from build123d import *

# Parameters (mm, degrees)
PAD_DEPTH       = 9.5
PAD001_DEPTH    = 9.5
SKETCH002_R     = 2.1
PAD002_DEPTH    = 3
POCKET_DEPTH    = 7
POCKET001_DEPTH = 7.3


with BuildPart() as part:
    # Sketch → Pad (new body, symmetric)
    with BuildSketch(Plane.YZ):
        Polygon((-9.4638496319, 12.9847787924), (0, 13.8127583485), (9.4638496319, 14.6407379046), (11.8731622478, 15.1748696522), (20.8002421453, 18.4240610138), (29.7273220428, 21.6732523754), (31.9162958532, 22.8127600156), (39.698240274, 28.2617361609), (47.4801846947, 33.7107123063), (49.7744904401, 30.4341041291), (34.2106015986, 19.5361518385), (31.0954026161, 17.9144818922), (13.2412428211, 11.416099169), (9.8124726029, 10.6559591122), (-9.1152266609, 9), (-12.6239030908, 9.1531921213), (-31.335250398, 12.452507497), (-34.6847225392, 13.5085920065), (-51.9045704929, 21.5383389795), (-50.2140974459, 25.1635701277), (-41.604173469, 21.1486966411), (-32.9942494922, 17.1338231546), (-30.6406576873, 16.391738509), (-21.2849840337, 14.7420808212), (-11.9293103801, 13.0924231333), align=None)
    extrude(amount=PAD_DEPTH, both=True)

    # Sketch001 → Pad001 (join)
    with BuildSketch(Plane.YZ):
        with BuildLine():
            Line((-32.3771396349, 6.543661009), (-30.6406576873, 16.391738509))
            Line((-30.6406576873, 16.391738509), (-32.9942494922, 17.1338231546))
            Line((-32.9942494922, 17.1338231546), (-37.2204319887, 8.0707452278))
            add(Edge.make_bspline(
                [(-37.2204319887, 8.0707452278), (-39.0096730727, 4.2337052069), (-40, 3), (-45, 3)],
                knots=[0, 0, 0, 0, 1, 1, 1, 1], degree=3))
            Line((-45, 3), (-45, 0))
            Line((-45, 0), (-35, 0))
            Line((-35, 0), (-32.3771396349, 6.543661009))
        make_face()
        Polygon((-13.6657925125, 3.2443456659), (-11.9293103801, 13.0924231333), (-9.4638496319, 12.9847787924), (-8.5922920505, 3.0228318249), (-8.5922920505, 0), (-13.6657925125, 0), align=None)
        Polygon((15.2933760081, 5.777947931), (11.8731622478, 15.1748696522), (9.4638496319, 14.6407379046), (10.3354072218, 4.6787909379), (10.3354072218, 0), (15.2933760081, 0), align=None)
        with BuildLine():
            Line((37.6520787719, 14.6212525652), (31.9162958532, 22.8127600156))
            Line((31.9162958532, 22.8127600156), (29.7273220428, 21.6732523754))
            Line((29.7273220428, 21.6732523754), (33.1475397634, 12.2763320956))
            Line((33.1475397634, 12.2763320956), (35, 0))
            Line((35, 0), (45, 0))
            Line((45, 0), (45, 2.9999999999))
            add(Edge.make_bspline(
                [(37.6520787719, 14.6212525652), (42.2621602037, 8.0374056988), (40, 2.999999954), (45, 2.9999999999)],
                knots=[0, 0, 0, 0, 1, 1, 1, 1], degree=3))
        make_face()
    extrude(amount=-PAD001_DEPTH)

    # Sketch002 → Pad002 (join)
    with BuildSketch(Plane.XY):
        with BuildLine():
            Line((0, -45), (-9.5, -45))
            Line((-9.5, -45), (-9.5, -55))
            Line((-9.5, -55), (4.5, -55))
            ThreePointArc((4.5, -55), (9.218348401, -51.6544450327), (7.6224992299, -46.0948753465))
            Line((0, -40), (7.6224992299, -46.0948753465))
            Line((0, -45), (0, -40))
        make_face()
        with Locations((0, -50)):
            Circle(SKETCH002_R, mode=Mode.SUBTRACT)
        with BuildLine():
            Line((0, 40), (0, 45))
            Line((0, 45), (-9.5, 45))
            Line((-9.5, 45), (-9.5, 55))
            Line((-9.5, 55), (4.5, 55))
            ThreePointArc((7.6224992299, 46.0948753465), (9.218348401, 51.6544450327), (4.5, 55))
            Line((7.6224992299, 46.0948753465), (0, 40))
        make_face()
        with Locations((0, 50)):
            Circle(SKETCH002_R, mode=Mode.SUBTRACT)
    extrude(amount=PAD002_DEPTH)

    # Sketch003 → Pocket (cut, symmetric)
    with BuildSketch(Plane.YZ):
        Polygon((-41.604173469, 21.1486966411), (-47.9483279783, 24.1070244733), (-48.540006161, 22.8381994546), (-49.718193731, 23.3875973412), (-50.8170011484, 21.0311970654), (-43.294646516, 17.523465493), (-35.7722918836, 14.0157339205), (-34.6734849555, 16.3721344244), (-35.85169762, 16.9215440128), (-35.2600189598, 18.190368809), align=None)
        Polygon((-28.1786383048, 15.9576180648), (-21.2849840337, 14.7420808212), (-14.3913297626, 13.5265435775), (-14.6344411843, 12.1478134238), (-13.3541878452, 11.922070218), (-13.8056723944, 9.3615699345), (-21.9795767444, 10.8028498091), (-30.1534810944, 12.2441296838), (-29.7019944172, 14.804629592), (-28.4217543468, 14.5788887258), align=None)
        Polygon((-6.9733628866, 13.2026681492), (0, 13.8127583484), (6.9733628866, 14.4228485476), (7.095382718, 13.0281761271), (8.3904355218, 13.141478566), (8.6170389651, 10.5513722208), (0.348622971, 9.8279795561), (-7.9197930232, 9.1045868913), (-8.1463876723, 11.6946940059), (-6.8513440135, 11.8079956448), align=None)
        Polygon((14.2223937998, 16.0299200105), (20.8002421453, 18.4240610138), (27.3780904908, 20.818202017), (27.8569247953, 19.5026345695), (29.078522765, 19.9472598688), (29.9677714711, 17.5040577202), (22.1683227186, 14.6652905306), (14.3688739661, 11.826523341), (13.4796328313, 14.2697282453), (14.7012277436, 14.7143524317), align=None)
        Polygon((33.964175964, 24.2467011065), (39.698240274, 28.2617361609), (45.432304584, 32.2767712154), (46.2353249737, 31.1299677214), (47.3002248466, 31.8756186398), (48.7915131317, 29.7458160079), (42.5661276004, 24.1659795418), (35.1935891965, 20.2244471644), (33.7022965595, 22.3542467491), (34.7671909619, 23.0998938371), align=None)
    extrude(amount=POCKET_DEPTH, both=True, mode=Mode.SUBTRACT)

    # Sketch004 → Pocket001 (cut, symmetric)
    with BuildSketch(Plane.YZ):
        Polygon((-48.4554802378, 23.0194599531), (-35.767171314, 17.1028043329), (-35.85169762, 16.9215440128), (-34.6734849555, 16.3721344244), (-35.0115879447, 15.6470921024), (-50.0562968731, 22.6625550904), (-49.718193731, 23.3875973412), (-48.540006161, 22.8381994546), align=None)
        Polygon((-29.7019944172, 14.804629592), (-29.8409228744, 14.0167851379), (-13.4931156588, 11.1342256504), (-13.3541878452, 11.922070218), (-14.6344411843, 12.1478134238), (-14.5997166858, 12.3447758803), (-28.3870287718, 14.7758509925), (-28.4217543468, 14.5788887258), align=None)
        Polygon((-6.8687714614, 12.0072349082), (-6.8513440135, 11.8079956448), (-8.1463876723, 11.6946940059), (-8.0766611038, 10.8977384201), (8.4601662766, 12.3445233466), (8.3904355218, 13.141478566), (7.095382718, 13.0281761271), (7.0779548525, 13.2274153539), align=None)
        Polygon((14.6328259169, 14.9022917574), (14.7012277436, 14.7143524317), (13.4796328313, 14.2697282453), (13.753251107, 13.5179749352), (29.3521455498, 19.1955081999), (29.078522765, 19.9472598688), (27.8569247953, 19.5026345695), (27.7885225257, 19.690573734), align=None)
        Polygon((34.7671909619, 23.0998938371), (33.7022965595, 22.3542467491), (34.1611654182, 21.698930512), (47.7590897918, 31.2202996624), (47.3002248466, 31.8756186398), (46.2353249737, 31.1299677214), (46.1206093491, 31.2937978941), (34.6524768556, 23.2637250729), align=None)
    extrude(amount=POCKET001_DEPTH, both=True, mode=Mode.SUBTRACT)


with BuildPart() as part_1:
    # Body placement: moved
    add(part.part.moved(Location((10, -10, 15))))


solid = part_1.part
Geometry: final body of the model. Coordinates: model frame, mm. A direction names the side the tool comes from. Round coordinates to 2 decimals unless told otherwise and drop trailing zeros. Order: outer loops, then holes, each group sorted by start corner. A loop starts at its lowest first (then second) coordinate and runs counter-clockwise, first axis right, second up. Notation, with made-up numbers: (29.5, 50) -> (75.5, 50) arc R22 cw to (75.5, 87) -> close; hole circle Ø10 at (58, 46). An arc over 180 degrees is marked (long way). Put each result on its own line as item: value. Start each with the question number.
Q1. Section B-B on x = 15.5. Give the number of separate pieces and of enclosed holes in the cut face, and give its area (3 significant figures).
Q2. First-contact query: pin 1 (6 mm diameter, centred on y = 3.5, z = 19, fed in from +X); pin 2 (1.5 mm diameter, centred on x = 16, y = 25.5, fed in from -Z); pin 3 (10 mm diameter, centred on x = 11.5, z = 39, fed in from +Y). Flat tips, straight axial feed; report the tip coordinate or a pass-through.
Q3. Section C-C on y = 13.5. Return the cut outline in (x, z), and give its area (3 significant figures).
Q4. Pull-direction query (Z, two-part tool) for faces 1 (the flat face through (3, -31, 29)), 2 (the flat face through (10.133, -41.834, 31.768)), 3 (the flat face through (14.82, 1.55, 26.04)), 4 (the flat face through (5.316, -18.857, 21.053)); classes: +Z half, -Z half, draft (parallel to the pull), parting line (faces both ways), or undercut.
Q5. Section A-A on y = -14.5. Return the cut outline in (x, z).
Q6. Reachability of faces 5 (the flat face through (2.7, -52.3, 34.8)), 6 (the flat face through (1.689, -9.868, 28.824)), 7 (the flat face through (9.9, -45.23, 30.18)) from +Z, -Z, +X, -X, +Y, -Y: full face, straight path, thin tool, end or side. Return the list, or none.
Q7. Line query: probe 1 along X at (y, z) = (-10.5, 26); probe 2 along Y at (x, z) = (6.75, 19); probe 3 along Y at (x, z) = (9.75, 17). Output: solid intervals per line, ascending.
Ans:
1. separate pieces: 8
1. enclosed holes: 0
1. area: 177 mm2
2. pin 1: stops at x = 10
2. pin 2: stops at z = 34.91
2. pin 3: stops at y = 25.19
3. outline: (0.5, 30.15) -> (3, 30.15) -> (3, 32.07) -> (2.7, 32.07) -> (2.7, 33.13) -> (3, 33.13) -> (3, 34.41) -> (0.5, 34.41) -> close; (17, 30.15) -> (19.5, 30.15) -> (19.5, 34.41) -> (17, 34.41) -> (17, 33.13) -> (17.3, 33.13) -> (17.3, 32.07) -> (17, 32.07) -> close
3. area: 20.6 mm2
4. face 1: draft
4. face 2: +Z half
4. face 3: -Z half
4. face 4: undercut
5. outline: (0.5, 24.4) -> (3, 24.4) -> (3, 26.21) -> (2.7, 26.21) -> (2.7, 27.21) -> (3, 27.21) -> (3, 28.42) -> (0.5, 28.42) -> close; (17, 24.4) -> (19.5, 24.4) -> (19.5, 28.42) -> (17, 28.42) -> (17, 27.21) -> (17.3, 27.21) -> (17.3, 26.21) -> (17, 26.21) -> close
6. face 5: none
6. face 6: +Z, +X, -X
6. face 7: -Y
7. probe 1: x = 0.5 to 3, 17 to 19.5
7. probe 2: y = -50.05 to -43.4, -23.53 to -18.68, 0.34 to 5.29, 24.4 to 32.29
7. probe 3: y = -65 to -62.09, -57.91 to -44.2, -23.67 to -18.59, 0.34 to 5.29, 24.7 to 37.91, 42.09 to 45
